Part model, mm, in its own coordinate system. Face numbers are marked on the shaded views. A direction names the side the tool comes from. Round coordinates to 2 decimals unless told otherwise and drop trailing zeros. Loops run counter-clockwise (first coordinate to the right, second up) from the corner with the lowest first, then second, coordinate; pieces in that order, holes last.
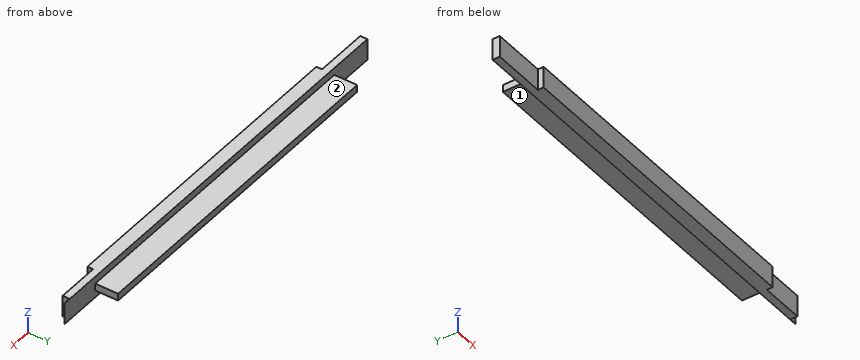
from build123d import *

# Parameters (mm, degrees)
SKETCH033_W     = 50
SKETCH033_H     = 30
PAD003_DEPTH    = 610
SKETCH034_W     = 70
SKETCH034_H     = 8
SKETCH034_W_2   = 60
SKETCH034_H_2   = 32
POCKET029_DEPTH = 30.001
SKETCH036_W     = 80
SKETCH036_H     = 32
SKETCH036_W_2   = 90
SKETCH036_H_2   = 8
POCKET031_DEPTH = 30.001
SKETCH037_W     = 32
SKETCH037_H     = 10
POCKET032_DEPTH = 1835.562096
SKETCH038_W     = 15
SKETCH038_H     = 50
POCKET033_DEPTH = 30.001
SKETCH039_W     = 10
SKETCH039_H     = 32.5
POCKET034_DEPTH = 30.001


with BuildPart() as part:
    # Sketch033 (on DatumPlane) → Pad003 (new body)
    with BuildSketch(Plane.YZ.offset(305)):
        Rectangle(SKETCH033_W, SKETCH033_H)
    extrude(amount=-PAD003_DEPTH)

    # Sketch034 (on DatumPlane) → Pocket029 (cut, through all)
    with BuildSketch(Plane.XY.offset(15)):
        with Locations((270, -21)):
            Rectangle(SKETCH034_W, SKETCH034_H)
        with Locations((275, 9)):
            Rectangle(SKETCH034_W_2, SKETCH034_H_2)
    extrude(amount=-POCKET029_DEPTH, mode=Mode.SUBTRACT)

    # Sketch036 (on DatumPlane) → Pocket031 (cut, through all)
    with BuildSketch(Plane.XY.offset(15)):
        with Locations((-265, 9)):
            Rectangle(SKETCH036_W, SKETCH036_H)
        with Locations((-260, -21)):
            Rectangle(SKETCH036_W_2, SKETCH036_H_2)
    extrude(amount=-POCKET031_DEPTH, mode=Mode.SUBTRACT)

    # Sketch037 (on DatumPlane) → Pocket032 (cut, through all)
    with BuildSketch(Plane.YZ.offset(305)):
        with Locations((9, 10)):
            Rectangle(SKETCH037_W, SKETCH037_H)
    pocket032 = extrude(amount=-POCKET032_DEPTH, mode=Mode.SUBTRACT)

    # Mirrored004: Pocket032 across Sketch037 H_Axis
    add(pocket032.mirror(Plane(origin=(305, 0, 0), x_dir=(1, 0, 0), z_dir=(0, 0, 1))), mode=Mode.SUBTRACT)

    # Sketch038 (on DatumPlane) → Pocket033 (cut, through all)
    with BuildSketch(Plane.XY.offset(15)):
        with Locations((-297.5, 0)):
            Rectangle(SKETCH038_W, SKETCH038_H)
    extrude(amount=-POCKET033_DEPTH, mode=Mode.SUBTRACT)

    # Sketch039 (on DatumPlane) → Pocket034 (cut, through all)
    with BuildSketch(Plane.XY.offset(15)):
        with Locations((300, -23.75)):
            Rectangle(SKETCH039_W, SKETCH039_H)
    extrude(amount=-POCKET034_DEPTH, mode=Mode.SUBTRACT)


solid = part.part
1) Wall check: line 1 along Y through (x, z) = (258.5, -6.25); line 2 along X through (y, z) = (-8.5, 12); line 3 along Y through (x, z) = (-75, 8.25). Give the ranges that are in metal, low to high.
Values:
line 1: y = -17 to -7
line 2: x = -290 to 295
line 3: y = -25 to -7
2) Slice it at C-C, the plane y = 12.5. Give the cut face in (x, z).
Values:
outline: (-225, -5) - (245, -5) - (245, 5) - (-225, 5) - close
3) Drop flat-ended pins along their axis: pin 1 Ø11 at (y, z) = (13.5, 1) entering from +X; pin 2 Ø9 at (x, z) = (265.5, -1.5) entering from -Y; pin 3 Ø3 at (x, z) = (302, 1) entering from -Y; pin 4 Ø8 at (y, z) = (18, -12) entering from +X. Give the stop position or say it passes through.
Values:
pin 1: stops at x = 245
pin 2: stops at y = -17
pin 3: stops at y = -7.5
pin 4: passes through
4) Slice it at A-A, the plane x = 6. Give the cut face in (y, z), then the cut area to 3 significant figures.
Values:
outline: (-25, -15) - (-7, -15) - (-7, -5) - (25, -5) - (25, 5) - (-7, 5) - (-7, 15) - (-25, 15) - close
area: 860 mm2
5) Slice it at B-B, the plane z = -10.5. Give the cut face in (x, y).
Values:
outline: (-290, -17) - (-215, -17) - (-215, -25) - (235, -25) - (235, -17) - (295, -17) - (295, -7.5) - (305, -7.5) - (305, -7) - (-290, -7) - close
6) Tool access for the marked faces 1 and 2: list every direction of +Z, -Z, +X, -X, +Y, -Y with a clear straight run to the whole face (end or side of a thin tool).
Values:
face 1: -Z, +X, -X, +Y
face 2: +Z, +X, -X, +Y
